Input: part model. Units: mm. Frame: model coordinates. A direction names the side the tool comes from. Round coordinates to 2 decimals unless told otherwise and drop trailing zeros. Loops run counter-clockwise (first coordinate to the right, second up) from the corner with the lowest first, then second, coordinate; pieces in that order, holes last. Notation, with made-up numbers: M 16,-21 L 21,-21 A20 cw 21,-3 Z; hole C 85.5,52 d9. An arc over 180 degrees is marked long. Return JSON: item names as keys, results as strings. Group by question number.
1) Access query for faces 1 (the face through (-19.05, -5, 82)), 2 (the face through (-1, 0, 45)). Directions: +Z, -Z, +X, -X, +Y, -Y. A direction counts if a zero-diameter tool reaches every point of the face in a straight line with its end or side. Return the directions, or none.
2) Contact query for flat-ended pins moving along their axis: P1, Ø1, axis at y = -1, z = 64, coming from the -X side (3 decimals); P2, Ø8.5, axis at x = 12.7, z = 83.17, coming from the -Y side; P3, Ø1.5, axis at y = -3, z = 18, coming from the -X side; P4, Ø3, axis at x = 6, y = -3, coming from the +Z side. Output: stop coordinate, or through.
3) Section A-A (x = 0). Output: boundary loops of the cut face in (y, z).
4) Section B-B (z = 57.15). Output: boundary loops of the cut face in (x, y), plus the area to 3 significant figures.
5) Material intervals for line 1 (X direction, y = -1.75, z = 83); line 2 (X direction, y = -8, z = 22); line 3 (X direction, y = -6.25, z = 19), sorted ascending. Write a range as from..to.
6) Mould query, pull axis Z, two halves, no side actions, for faces 3 (the face through (-13.388, -4.93, 80.074)), 4 (the face through (-60.97, -7.583, 17.952)), 5 (the face through (-62.04, -4.93, 49.51)), 6 (the face through (19.05, -5, 82)). Classes: +Z half, -Z half, draft (parallel to the pull), parting line (faces both ways), or undercut.
from build123d import *

# Parameters (mm, degrees)
F2_R     = 6.5
F2_R_2   = 3.175
F3_DEPTH = 10
F0_SIZE  = 5.08
F1_SIZE  = 2.54


# Not quite as in the source:
# - a feature names something its author has since deleted; it is built from what else it names


with BuildPart() as f3:
    # F2 (on Front) → F3 (new body)
    with BuildSketch(Plane.XZ):
        with BuildLine():
            Line((-19.05, 86.834944003), (-19.05, 77.0550979819))
            ThreePointArc((-19.05, 77.0550979819), (-62.4999375, 48.9300361486), (-79.375, 0))
            Line((-79.375, 0), (-28.25, 0))
            ThreePointArc((-28.25, 0), (0, 28.25), (28.25, 0))
            Line((28.25, 0), (79.375, 0))
            ThreePointArc((79.375, 0), (62.4999375, 48.9300361486), (19.05, 77.0550979819))
            Line((19.05, 77.0550979819), (19.05, 86.834944003))
            ThreePointArc((19.05, 86.834944003), (0, 88.9), (-19.05, 86.834944003))
        make_face()
        with Locations((-54.3528799063, 17.6603212285)):
            Circle(F2_R, mode=Mode.SUBTRACT)
        with Locations((54.3528799063, 17.6603212285)):
            Circle(F2_R, mode=Mode.SUBTRACT)
        with Locations((-12.7, 83.1734867987)):
            Circle(F2_R_2, mode=Mode.SUBTRACT)
        with Locations((0, 57.15)):
            Circle(F2_R, mode=Mode.SUBTRACT)
        with Locations((12.7, 83.1734867987)):
            Circle(F2_R_2, mode=Mode.SUBTRACT)
    extrude(amount=F3_DEPTH)

    # F0
    f0_edges = [f3.edges().sort_by_distance(p)[0] for p in [
        (0, -10, 28.25),
    ]]
    chamfer(f0_edges, length=F0_SIZE)

    # F1
    f1_edges = [f3.edges().sort_by_distance(p)[0] for p in [
        (-6.5, -10, 57.15),
        (-60.85288, -10, 17.660321),
        (47.85288, -10, 17.660321),
    ]]
    chamfer(f1_edges, length=F1_SIZE)


solid = f3.part
Returned:
{
 "1": {"face 1": "+Z, -X, +Y, -Y", "face 2": "+Z, -Z, +X, -X, +Y"},
 "2": {"P1": "stops at x = -47.625", "P2": "stops at y = -10", "P3": "stops at x = -77.48", "P4": "stops at z = 88.79"},
 "3": {"outline": "M -10,33.33 L -4.92,28.25 L 0,28.25 L 0,50.65 L -7.46,50.65 L -10,48.11 Z; M -10,66.19 L -7.46,63.65 L 0,63.65 L 0,88.9 L -10,88.9 Z"},
 "4": {"outline": "M -55.08,-10 L -9.04,-10 L -6.5,-7.46 L -6.5,0 L -55.08,0 Z; M 6.5,-7.46 L 9.04,-10 L 55.08,-10 L 55.08,0 L 6.5,0 Z", "area": "965 mm^2"},
 "5": {"line 1": "x = -19.05..-15.87, -9.53..9.53, 15.87..19.05", "line 2": "x = -76.27..-59.9, -48.81..-22.31, 22.31..48.81, 59.9..76.27", "line 3": "x = -77.07..-60.71, -47.99..-22.67, 22.67..47.99, 60.71..77.07"},
 "6": {"face 3": "undercut", "face 4": "undercut", "face 5": "+Z half", "face 6": "draft"}
}
